Input: dimensioned drawing with shaded views. Units: mm. Origin: part minimum x, y, z. Coordinates: 2 decimals unless noted, no trailing zeros. Write each loop counter-clockwise with the first axis right and the second up, starting at its lowest first coordinate (ties: lowest second). Pieces come first, ordered by that corner, then holes. Notation, with made-up numbers: M 24.5,0.5 L 43.5,0.5 A14 cw 43.5,4.5 Z; hole C -7,19 d11. An arc over 180 degrees is marked long. Use one line per item in the form item = value.
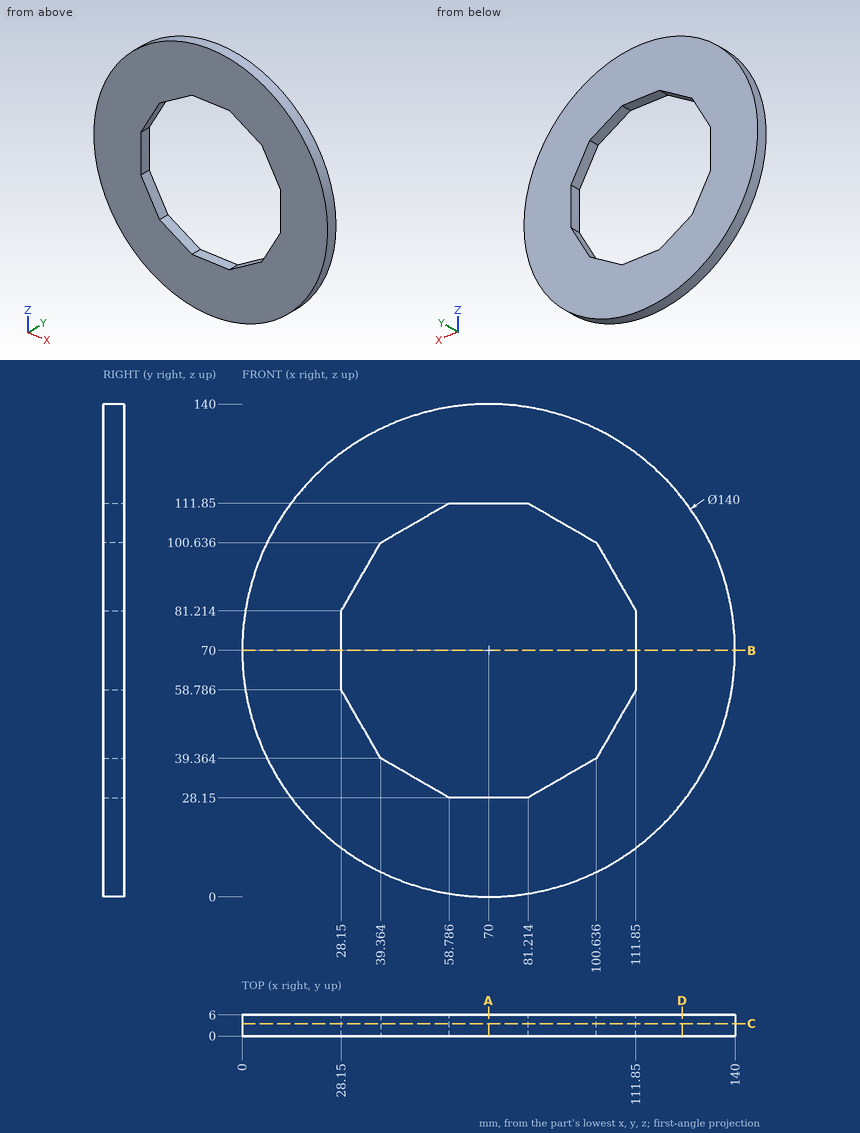
(1) First-contact query: pin 1 Ø1.8 at (y, z) = (3.5, 74) entering from -X; pin 2 Ø2 at (x, y) = (112, 4) entering from -Z; pin 3 Ø1.8 at (x, y) = (74, 4) entering from +Z. Flat tips, straight axial feed; report the tip coordinate or a pass-through.
Computed:
pin_1 = 0.07
pin_2 = 13.26
pin_3 = 139.93
(2) Section query A-A on x = 70. Return the cut outline in (y, z).
Computed:
outline = M 0,0 L 6,0 L 6,28.15 L 0,28.15 Z; M 0,111.85 L 6,111.85 L 6,140 L 0,140 Z
(3) Section query D-D on x = 125. Return the cut outline in (y, z).
Computed:
outline = M 0,26.7 L 6,26.7 L 6,113.3 L 0,113.3 Z
(4) Section query C-C on y = 3.5. Return the cut outline in (x, z), plus the area to 3 significant figures.
Computed:
outline = C 70,70 d140; hole M 28.15,58.79 L 39.36,39.36 L 58.79,28.15 L 81.21,28.15 L 100.64,39.36 L 111.85,58.79 L 111.85,81.21 L 100.64,100.64 L 81.21,111.85 L 58.79,111.85 L 39.36,100.64 L 28.15,81.21 Z
area = 9,760 mm^2
(5) Line query: probe 1 along Z at (x, y) = (69, 2.9); probe 2 along Z at (x, y) = (31.5, 2.15) (1 decimal); probe 3 along X at (y, z) = (3.9, 96). Output: solid intervals per line, ascending.
Computed:
probe_1 = 0.01 to 28.15, 111.85 to 139.99
probe_2 = 11.5 to 53, 87 to 128.5
probe_3 = 5.01 to 36.69, 103.31 to 134.99
(6) Section query B-B on z = 70. Return the cut outline in (x, y).
Computed:
outline = M 0,0 L 28.15,0 L 28.15,6 L 0,6 Z; M 111.85,0 L 140,0 L 140,6 L 111.85,6 Z
